Work out the finished part from the listing and answer in its coordinate system (mm). A direction names the side the tool comes from. Round coordinates to 2 decimals unless told otherwise and drop trailing zeros. Loops run counter-clockwise (first coordinate to the right, second up) from the corner with the lowest first, then second, coordinate; pieces in that order, holes last. Notation, with made-up numbers: M 59,38 L 113,38 A31 ccw 113,76 Z; hole C -35.75,33 d3. An arc over 180 degrees is marked long. One line per item, written item: value.
```python
from build123d import *

# Parameters (mm, degrees)
BOSS_EXTRUDE1_DEPTH            = 45
CBORE_FOR_M3_SHCS1_D           = 3.2
CBORE_FOR_M3_SHCS1_CBORE_D     = 6.5
CBORE_FOR_M3_SHCS1_CBORE_DEPTH = 3
F_25_0_25_DIAMETER_HOLE1_D     = 25
CHAMFER1_SIZE                  = 1
M3X0_5_TAPPED_HOLE1_D          = 2.5
M3X0_5_TAPPED_HOLE1_DEPTH      = 7.5
M3X0_5_TAPPED_HOLE1_TIP        = 0.751075774
F_3_0MM_DOWEL_HOLE1_D          = 3
F_3_0MM_DOWEL_HOLE1_DEPTH      = 7.5
F_3_0MM_DOWEL_HOLE1_TIP        = 0.901290929


with BuildPart() as part:
    # Sketch1 → Boss-Extrude1 (new body)
    with BuildSketch(Plane.XY):
        Polygon((3.23, 30.362745098), (3.23, 22.362745098), (0, 22.362745098), (0, -15.637254902), (7, -15.637254902), (7, 30.362745098), align=None)
    extrude(amount=BOSS_EXTRUDE1_DEPTH)

    # CBORE for M3 SHCS1 (through all)
    with Locations(Plane(origin=(7, 0, 0), x_dir=(0, 0, -1), z_dir=(1, 0, 0))):
        with Locations((-20, 26.362745098)):
            CounterBoreHole(CBORE_FOR_M3_SHCS1_D / 2, CBORE_FOR_M3_SHCS1_CBORE_D / 2, CBORE_FOR_M3_SHCS1_CBORE_DEPTH)

    # Ø25.0 (25) Diameter Hole1 (through all)
    with Locations(Plane(origin=(7, 0, 0), x_dir=(0, 0, -1), z_dir=(1, 0, 0))):
        with Locations((-20, 4.362745098)):
            Hole(F_25_0_25_DIAMETER_HOLE1_D / 2)

    # Chamfer1
    # the kernel refuses this chamfer: 1 mm, written as the material it takes off along each edge
    with BuildSketch(Plane(origin=(7, 30.362745098, -2.571682988), x_dir=(-0.9996219169112968, 0.027495876610585623, 0), z_dir=(0, 0, 1))) as chamfer1_piece_1:
        Polygon((CHAMFER1_SIZE * 0.999621916911, CHAMFER1_SIZE * 0.0274958766106), (-CHAMFER1_SIZE * 0.0274958766106, CHAMFER1_SIZE * 0.999621916911), (0, 0), align=None)
    extrude(amount=50.143365976, mode=Mode.SUBTRACT)

    # M3x0.5 Tapped Hole1
    with Locations(Plane(origin=(0, -15.637254902, 0), x_dir=(-1, 0, 0), z_dir=(0, -1, 0))):
        with Locations((-3.5, -24)):
            Hole(M3X0_5_TAPPED_HOLE1_D / 2, depth=M3X0_5_TAPPED_HOLE1_DEPTH)
            with Locations((0, 0, -(M3X0_5_TAPPED_HOLE1_DEPTH + M3X0_5_TAPPED_HOLE1_TIP / 2))):  # 118° drill point
                Cone(0, M3X0_5_TAPPED_HOLE1_D / 2, M3X0_5_TAPPED_HOLE1_TIP, mode=Mode.SUBTRACT)

    # Ø3.0mm Dowel Hole1
    with Locations(Plane(origin=(0, -15.637254902, 0), x_dir=(-1, 0, 0), z_dir=(0, -1, 0))):
        with Locations((-3.5, -38), (-3.5, -7)):
            Hole(F_3_0MM_DOWEL_HOLE1_D / 2, depth=F_3_0MM_DOWEL_HOLE1_DEPTH)
            with Locations((0, 0, -(F_3_0MM_DOWEL_HOLE1_DEPTH + F_3_0MM_DOWEL_HOLE1_TIP / 2))):  # 118° drill point
                Cone(0, F_3_0MM_DOWEL_HOLE1_D / 2, F_3_0MM_DOWEL_HOLE1_TIP, mode=Mode.SUBTRACT)


solid = part.part
```
1) Find section A-A (z = 41). Give the vertices of the cut face in (x, y).
Check values:
outline: M 0,-15.64 L 7,-15.64 L 7,29.36 L 6,30.36 L 3.23,30.36 L 3.23,22.36 L 0,22.36 Z
2) The mould has two halves that part along Z. Classify faces 1 (the face through (3, 8, 0)), 2 (the face through (0, -1, 32)), 3 (the face through (3, 8, 45)), 4 (the face through (3.534, -7.392, 37.742)): +Z half, -Z half, draft (parallel to the pull), parting line (faces both ways), or undercut.
Check values:
face 1: -Z half
face 2: draft
face 3: +Z half
face 4: undercut
3) For faces 5 (the face through (4.19, -11.83, 39.33)), 6 (the face through (4, 28, 19)), 7 (the face through (3.23, 26, 22)), determine the directions among +Z, -Z, +X, -X, +Y, -Y from which every point of the face is accessible in a straight line to the end or side of a thin tool.
Check values:
face 5: -Y
face 6: +X
face 7: +Z, -Z, -X, +Y
4) Find section D-D (z = 14). Give the vertices of the cut face in (x, y).
Check values:
outline: M 0,-15.64 L 7,-15.64 L 7,-6.6 L 0,-6.6 Z; M 0,15.33 L 7,15.33 L 7,29.36 L 6,30.36 L 3.23,30.36 L 3.23,22.36 L 0,22.36 Z
5) Find section C-C (z = 20). Give the vertices of the cut face in (x, y), then the cut area to 3 significant figures.
Check values:
outline: M 0,-15.64 L 7,-15.64 L 7,-8.14 L 0,-8.14 Z; M 0,16.86 L 7,16.86 L 7,23.11 L 4,23.11 L 4,24.76 L 3.23,24.76 L 3.23,22.36 L 0,22.36 Z; M 3.23,27.96 L 4,27.96 L 4,29.61 L 6.75,29.61 L 6,30.36 L 3.23,30.36 Z
area: 98.7 mm2
6) Each of these flat-tipped pins is pushed along its axis until it touches: pin 1 (1.8 mm diameter, centred on x = 3.5, z = 38, fed in from -Y); pin 2 (5 mm diameter, centred on y = 26.36, z = 20, fed in from -X); pin 3 (3 mm diameter, centred on y = 26.5, z = 18.5, fed in from +X). Where does it stop, or does it pass through?
Check values:
pin 1: y = -7.78
pin 2: x = 3.23
pin 3: x = 4
7) Find section B-B (y = -3). Give the vertices of the cut face in (x, z).
Check values:
outline: M 0,0 L 7,0 L 7,9.9 L 0,9.9 Z; M 0,30.1 L 7,30.1 L 7,45 L 0,45 Z
8) Find the intervals of material crossed by probe 1 along Y at (x, z) = (5.85, 20); probe 2 along Y at (x, z) = (3.7, 20); probe 3 along Z at (x, y) = (3.5, -10), in increasing order. Write a range as from..to.
Check values:
probe 1: -15.64..-8.14, 16.86..23.11, 29.61..30.36
probe 2: -15.64..-8.14, 16.86..24.76, 27.96..30.36
probe 3: 0..5.5, 8.5..22.75, 25.25..36.5, 39.5..45
